Source: CAD feature listing. Evaluate the final solid. Frame: model axes, mm. A direction names the side the tool comes from. Coordinates: 2 decimals unless noted, no trailing zeros. Loops run counter-clockwise (first coordinate to the right, second up) from the corner with the lowest first, then second, coordinate; pieces in that order, holes last.
from build123d import *

# Parameters (mm, degrees)
BOSS_EXTRUDE5_DEPTH      = 25
BOSS_EXTRUDE5_2_DEPTH    = 25
BOSS_EXTRUDE5_3_DEPTH    = 25
BOSS_EXTRUDE5_4_DEPTH    = 25
SKETCH5_R                = 97.102354857
SKETCH5_R_2              = 87.102354857
BOSS_EXTRUDE6_DEPTH      = 2100
BOSS_EXTRUDE6_DEPTH_BACK = 273


with BuildPart() as part:
    # Sketch4 → Boss-Extrude5 (new body)
    with BuildSketch(Plane.XY):
        with BuildLine():
            Line((-283.528917558, -59.677513544), (-95.020352129, -20))
            ThreePointArc((-95.020352129, -20), (-97.102354857, 0), (-95.020352129, 20))
            Line((-95.020352129, 20), (-283.528917558, 59.677513544))
            ThreePointArc((-283.528917558, 59.677513544), (-289.741354857, 0), (-283.528917558, -59.677513544))
        make_face()
        with BuildLine():
            ThreePointArc((-103.749908429, 11.618296452), (-100.811412037, 0.266569794), (-102.448791191, -11.344435703))
            Line((-102.448791191, -11.344435703), (-263.440278466, -40.343403868))
            ThreePointArc((-263.440278466, -40.343403868), (-268.408850648, 0.533483895), (-260.728236447, 40.988580338))
            Line((-260.728236447, 40.988580338), (-103.749908429, 11.618296452))
        make_face(mode=Mode.SUBTRACT)
    extrude(amount=BOSS_EXTRUDE5_DEPTH)



with BuildPart() as body_2:
    # Sketch4 → Boss-Extrude5 2 (new body)
    with BuildSketch(Plane.XY):
        with BuildLine():
            Line((-59.677513544, 283.528917558), (-20, 95.020352129))
            ThreePointArc((-20, 95.020352129), (0, 97.102354857), (20, 95.020352129))
            Line((20, 95.020352129), (59.677513544, 283.528917558))
            ThreePointArc((59.677513544, 283.528917558), (0, 289.741354857), (-59.677513544, 283.528917558))
        make_face()
        with BuildLine():
            Line((40.988580338, 260.728236447), (11.618296452, 103.749908429))
            ThreePointArc((11.618296452, 103.749908429), (0.266569794, 100.811412037), (-11.344435703, 102.448791191))
            Line((-11.344435703, 102.448791191), (-40.343403868, 263.440278466))
            ThreePointArc((-40.343403868, 263.440278466), (0.533483895, 268.408850648), (40.988580338, 260.728236447))
        make_face(mode=Mode.SUBTRACT)
    extrude(amount=BOSS_EXTRUDE5_2_DEPTH)


with BuildPart() as body_3:
    # Sketch4 → Boss-Extrude5 3 (new body)
    with BuildSketch(Plane.XY):
        with BuildLine():
            ThreePointArc((97.102354857, 0), (96.580451619, -10.054038186), (95.020352129, -20))
            Line((95.020352129, -20), (283.528917558, -59.677513544))
            ThreePointArc((283.528917558, -59.677513544), (289.741354857, 0), (283.528917558, 59.677513544))
            Line((283.528917558, 59.677513544), (95.020352129, 20))
            ThreePointArc((95.020352129, 20), (96.580451619, 10.054038186), (97.102354857, 0))
        make_face()
        with BuildLine():
            Line((260.728236447, -40.988580338), (103.749908429, -11.618296452))
            ThreePointArc((103.749908429, -11.618296452), (100.811412037, -0.266569794), (102.448791191, 11.344435703))
            Line((102.448791191, 11.344435703), (263.440278466, 40.343403868))
            ThreePointArc((263.440278466, 40.343403868), (268.408850648, -0.533483895), (260.728236447, -40.988580338))
        make_face(mode=Mode.SUBTRACT)
    extrude(amount=BOSS_EXTRUDE5_3_DEPTH)


with BuildPart() as body_4:
    # Sketch4 → Boss-Extrude5 4 (new body)
    with BuildSketch(Plane.XY):
        with BuildLine():
            ThreePointArc((20, -95.020352129), (0, -97.102354857), (-20, -95.020352129))
            Line((-20, -95.020352129), (-59.677513544, -283.528917558))
            ThreePointArc((-59.677513544, -283.528917558), (0, -289.741354857), (59.677513544, -283.528917558))
            Line((59.677513544, -283.528917558), (20, -95.020352129))
        make_face()
        with BuildLine():
            Line((-40.988580338, -260.728236447), (-11.618296452, -103.749908429))
            ThreePointArc((-11.618296452, -103.749908429), (-0.266569794, -100.811412037), (11.344435703, -102.448791191))
            Line((11.344435703, -102.448791191), (40.343403868, -263.440278466))
            ThreePointArc((40.343403868, -263.440278466), (-0.533483895, -268.408850648), (-40.988580338, -260.728236447))
        make_face(mode=Mode.SUBTRACT)
    extrude(amount=BOSS_EXTRUDE5_4_DEPTH)


with BuildPart() as part_1:
    add(part.part)

    add(body_2.part)  # Boss-Extrude6 merges body 2

    add(body_3.part)  # Boss-Extrude6 merges body 3

    add(body_4.part)  # Boss-Extrude6 merges body 4
    # Sketch5 → Boss-Extrude6 (add, two sides)
    with BuildSketch(Plane.XY) as boss_extrude6_sk:
        Circle(SKETCH5_R)
        Circle(SKETCH5_R_2, mode=Mode.SUBTRACT)
    extrude(amount=BOSS_EXTRUDE6_DEPTH)
    extrude(boss_extrude6_sk.sketch, amount=-BOSS_EXTRUDE6_DEPTH_BACK)


solid = part_1.part
Q1. Section B-B, the plane x = 189. Return the cut outline in (y, z).
Q2. Line query: line 1 along Y through (x, z) = (0, -81); line 2 along X through (y, z) = (-33, 1679); line 3 along X through (y, z) = (-77, 366.5). Output: solid intervals per line, ascending.
Q3. Access query for faces 1 (the flat face through (-39.561, -187.955, 12.325)), 2 (the flat face through (40.116, -190.594, 12.325)), 3 (the flat face through (-190.594, -40.116, 12.325)), 4 (the flat face through (-187.955, 39.561, 12.325)). Directions: +Z, -Z, +X, -X, +Y, -Y. A direction counts if a zero-diameter tool reaches every point of the face in a straight line with its end or side. Return the directions, or none.
Q4. Section A-A, the plane y = 130. Return the cut outline in (x, z), plus the area to 3 significant figures.
Q5. Draft query along X for faces 5 (the flat face through (-36, 80, 2100)), 6 (the flat face through (190.594, 40.116, 12.325)), 7 (the flat face through (39.561, 187.955, 12.325)). Return one class per face: +X half, -X half, draft (parallel to the pull), parting line (faces both ways), or undercut.
Q6. Section C-C, the plane z = 1283. Return the cut outline in (x, y).
Q7. Contact query for flat-ended pins moving along their axis: pin 1 Ø1.5 at (x, z) = (13.5, 54.5) entering from -Y; pin 2 Ø12 at (x, y) = (-32.5, -165.5) entering from -Z; pin 3 Ø8 at (x, z) = (-53, 1525) entering from -Y. Output: stop coordinate, or through.
Derived:
1. outline: (-39.78, 0) - (-27.57, 0) - (-27.57, 25) - (-39.78, 25) - close; (26.93, 0) - (39.78, 0) - (39.78, 25) - (26.93, 25) - close
2. line 1: y = -97.1 to -87.1, 87.1 to 97.1
2. line 2: x = -91.32 to -80.61, 80.61 to 91.32
2. line 3: x = -59.16 to -40.72, 40.72 to 59.16
3. face 1: +Z, -Z, -X
3. face 2: +Z, -Z, +X
3. face 3: +Z, -Z, -Y
3. face 4: +Z, -Z, +Y
4. outline: (-27.36, 0) - (-16.31, 0) - (-16.31, 25) - (-27.36, 25) - close; (16.53, 0) - (27.36, 0) - (27.36, 25) - (16.53, 25) - close
4. area: 547 mm2
5. face 5: draft
5. face 6: undercut
5. face 7: +X half
6. outline: circle Ø194.2 at (0, 0); hole circle Ø174.2 at (0, 0)
7. pin 1: stops at y = -96.26
7. pin 2: stops at z = 0
7. pin 3: stops at y = -83.83
